```python
from build123d import *

# Parameters (mm, degrees)
SKETCH1_R           = 12
BOSS_EXTRUDE1_DEPTH = 1.2
SKETCH2_R           = 6.25
BOSS_EXTRUDE2_DEPTH = 13.8
SKETCH3_R           = 2.5
BOSS_EXTRUDE3_DEPTH = 1.5
SKETCH4_R           = 1.6
CUT_EXTRUDE1_DEPTH  = 1.2


with BuildPart() as part:
    # Sketch1 → Boss-Extrude1 (new body)
    with BuildSketch(Plane(origin=(0, 0, 0), x_dir=(1, 0, 0), z_dir=(0, 1, 0))):
        with Locations(Location((0, 0, 0), (0, 0, 270))):
            Circle(SKETCH1_R)
    extrude(amount=BOSS_EXTRUDE1_DEPTH)

    # Sketch2 → Boss-Extrude2 (add)
    with BuildSketch(Plane(origin=(0, 1.2, 0), x_dir=(1, 0, 0), z_dir=(0, 1, 0))):
        with Locations(Location((0, 0, 0), (0, 0, 90))):
            Circle(SKETCH2_R)
    extrude(amount=BOSS_EXTRUDE2_DEPTH)

    # Sketch3 → Boss-Extrude3 (add)
    with BuildSketch(Plane.XZ):
        with Locations(Location((0, 0, 0), (0, 0, 270))):
            Circle(SKETCH3_R)
    extrude(amount=BOSS_EXTRUDE3_DEPTH)

    # Sketch4 → Cut-Extrude1 (cut)
    with BuildSketch(Plane.XZ):
        with Locations(Location((0, 9, 0), (0, 0, 270))):
            Circle(SKETCH4_R)
        with Locations(Location((7.794228634, -4.5, 0), (0, 0, 270))):
            Circle(SKETCH4_R)
        with Locations(Location((-7.794228634, -4.5, 0), (0, 0, 270))):
            Circle(SKETCH4_R)
    extrude(amount=-CUT_EXTRUDE1_DEPTH, mode=Mode.SUBTRACT)


solid = part.part
```
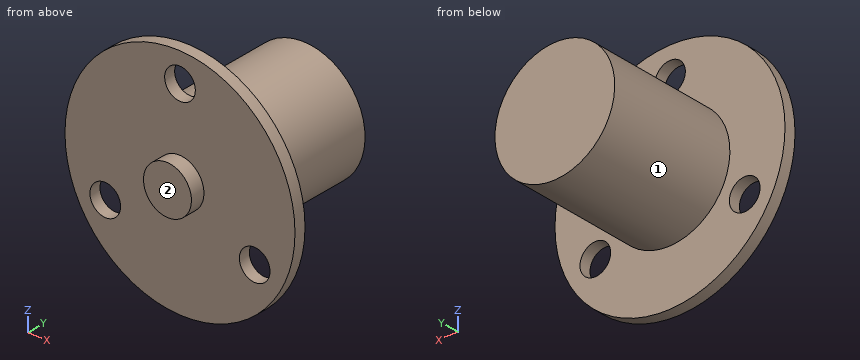
Here's how the part is built. I have some questions about the finished solid (model axes, mm). Face numbers are marked on the shaded views. A direction names the side the tool comes from. Give positions to 0.01 mm unless a question says otherwise; leave off trailing zeros. Order: outer loops, then holes, each group sorted by start corner. A loop starts at its lowest first (then second) coordinate and runs counter-clockwise, first axis right, second up. Notation, with made-up numbers: (-31, -38) -> (13, -38) arc R31 cw to (13, -9) -> close; hole circle Ø3 at (-37.5, 62.25). An arc over 180 degrees is marked (long way). Use CSV: the item, a comma, the result in double quotes. Start each with the question number.
Item 1: Suppose I cut it at A-A (x = 0). List the corners of the cut face in (y, z) for me.
Item 2: On a 3-axis mill with a long thin cutter (end or side, diameter ignored), from which of +Z, -Z, +X, -X, +Y, -Y can I reach the whole of each face in a straight line? I mean the marked faces 1 and 2. Say none if no direction works.
Item 3: I'm going to push flat-ended pins straight in: P1, Ø5, axis at x = 7.79, z = -4.5, coming from the -Y side; P2, Ø3, axis at x = -7.79, z = -4.5, coming from the +Y side; P3, Ø3, axis at y = 7, z = -2, coming from the -X side; P4, Ø3, axis at x = -5, z = -4, coming from the +Y side. Where does each tip first touch, or does it pass through?
Item 4: Suppose I cut it at B-B (z = 10.25). List the corners of the cut face in (x, y) for me.
Item 5: Suppose I cut it at C-C (z = -4.5). List the corners of the cut face in (x, y) for me.
Item 6: If I drill on probe 1 along X at (y, z) = (0.55, -4.5); probe 2 along Y at (x, z) = (2.5, -6); probe 3 along Y at (x, z) = (-2.25, 2.25), over which ranges is the centre line in solid material (lowest first)? Write a range as [from, to].
Item 7: Suppose I cut it at D-D (y = 11). List the corners of the cut face in (x, z) for me.
Answer block:
1,outline,"(-1.5, -2.5) -> (0, -2.5) -> (0, -12) -> (1.2, -12) -> (1.2, -6.25) -> (15, -6.25) -> (15, 6.25) -> (1.2, 6.25) -> (1.2, 7.4) -> (0, 7.4) -> (0, 2.5) -> (-1.5, 2.5) -> close; (0, 10.6) -> (1.2, 10.6) -> (1.2, 12) -> (0, 12) -> close"
2,face 1,"+Y"
2,face 2,"+Z, -Z, +X, -X, -Y"
3,P1,"stops at y = 0"
3,P2,"passes through"
3,P3,"stops at x = -6.23"
3,P4,"stops at y = 15"
4,outline,"(-6.24, 0) -> (-1, 0) -> (-1, 1.2) -> (-6.24, 1.2) -> close; (1, 0) -> (6.24, 0) -> (6.24, 1.2) -> (1, 1.2) -> close"
5,outline,"(-11.12, 0) -> (-9.39, 0) -> (-9.39, 1.2) -> (-11.12, 1.2) -> close; (-6.19, 0) -> (6.19, 0) -> (6.19, 1.2) -> (4.34, 1.2) -> (4.34, 15) -> (-4.34, 15) -> (-4.34, 1.2) -> (-6.19, 1.2) -> close; (9.39, 0) -> (11.12, 0) -> (11.12, 1.2) -> (9.39, 1.2) -> close"
6,probe 1,"x = [-11.12, -9.39], [-6.19, 6.19], [9.39, 11.12]"
6,probe 2,"y = [0, 1.2]"
6,probe 3,"y = [0, 15]"
7,outline,"circle Ø12.5 at (0, 0)"
